```python
from build123d import *

# Parameters (mm, degrees)
F1_DEPTH = 0.5


# Not quite as in the source:
# - a pattern or mirror of a feature is missing from the dataset's text; its kind, count and spacing are read off the source's solid


with BuildPart() as f1:
    # F0 (on Top) → F1 (new body)
    with BuildSketch(Plane.XY):
        Polygon((160, 0), (0, 0), (0, -1), (0, -160), (160, -160), align=None)
        Polygon((1, -1.7071067812), (1, -1), (1.7071067812, -1), (79.5, -1), (80, -1), (80.5, -1), (158.2928932188, -1), (159, -1), (159, -1.7071067812), (159, -79.5), (159, -80.5), (159, -158.2928932188), (159, -159), (158.2928932188, -159), (80.5, -159), (80, -159), (79.5, -159), (1.7071067812, -159), (1, -159), (1, -158.2928932188), (1, -80.5), (1, -80), (1, -79.5), align=None, mode=Mode.SUBTRACT)
        Polygon((78.7928932188, -79.5), (1, -79.5), (1, -80), (1, -80.5), (78.7928932188, -80.5), (79.2928932188, -80), align=None)
        Polygon((159, -79.5), (81.2071067812, -79.5), (80.7071067812, -80), (81.2071067812, -80.5), (159, -80.5), align=None)
        Polygon((79.5, -78.7928932188), (1.7071067812, -1), (1.3535533906, -1.3535533906), (79.5, -79.5), align=None)
        Polygon((1.3535533906, -1.3535533906), (1, -1.7071067812), (78.7928932188, -79.5), (79.5, -79.5), align=None)
        Polygon((146.2407427602, -146.2407427602), (80.5, -80.5), (80.5, -81.2071067812), (145.8871893697, -146.5942961508), align=None)
        Polygon((81.2071067812, -80.5), (80.5, -80.5), (146.2407427602, -146.2407427602), (146.5942961508, -145.8871893697), align=None)
        Polygon((80, -1), (79.5, -1), (79.5, -78.7928932188), (80, -79.2928932188), align=None)
        Polygon((80.5, -1), (80, -1), (80, -79.2928932188), (80.5, -78.7928932188), align=None)
        Polygon((80, -80.7071067812), (79.5, -81.2071067812), (79.5, -159), (80, -159), align=None)
        Polygon((80.5, -81.2071067812), (80, -80.7071067812), (80, -159), (80.5, -159), align=None)
        Polygon((146.5942961508, -145.8871893697), (146.2407427602, -146.2407427602), (158.6464466094, -158.6464466094), (159, -158.2928932188), align=None)
        Polygon((158.6464466094, -158.6464466094), (146.2407427602, -146.2407427602), (145.8871893697, -146.5942961508), (158.2928932188, -159), align=None)
        Polygon((159, -1), (158.2928932188, -1), (149.7961722435, -9.4967209753), (150.1497256341, -9.8502743659), align=None)
        Polygon((159, -1.7071067812), (159, -1), (150.1497256341, -9.8502743659), (150.5032790247, -10.2038277565), align=None)
        Polygon((80, -79.2928932188), (79.5, -78.7928932188), (79.5, -79.5), (79.7928932188, -79.5), align=None)
        Polygon((79.5, -79.5), (78.7928932188, -79.5), (79.2928932188, -80), (79.5, -79.7928932188), align=None)
        Polygon((80.5, -78.7928932188), (80, -79.2928932188), (80.2071067812, -79.5), (80.5, -79.5), align=None)
        Polygon((79.5, -80.2071067812), (79.2928932188, -80), (78.7928932188, -80.5), (79.5, -80.5), align=None)
        Polygon((80, -80), (79.6464466094, -79.6464466094), (79.5, -79.7928932188), (79.5, -80.2071067812), (79.6464466094, -80.3535533906), align=None)
        Polygon((80.3535533906, -79.6464466094), (80, -80), (80.3535533906, -80.3535533906), (80.5, -80.2071067812), (80.5, -79.7928932188), align=None)
        Polygon((81.2071067812, -79.5), (80.5, -79.5), (80.5, -79.7928932188), (80.7071067812, -80), align=None)
        Polygon((79.7928932188, -80.5), (79.5, -80.5), (79.5, -81.2071067812), (80, -80.7071067812), align=None)
        Polygon((80.5, -80.5), (80.2071067812, -80.5), (80, -80.7071067812), (80.5, -81.2071067812), align=None)
        Polygon((80.7071067812, -80), (80.5, -80.2071067812), (80.5, -80.5), (81.2071067812, -80.5), align=None)
        Polygon((1.7071067812, -1), (1, -1), (1.3535533906, -1.3535533906), align=None)
        Polygon((1.3535533906, -1.3535533906), (1, -1), (1, -1.7071067812), align=None)
        Polygon((1.3535533906, -158.6464466094), (1, -158.2928932188), (1, -159), align=None)
        Polygon((1.3535533906, -158.6464466094), (1, -159), (1.7071067812, -159), align=None)
        Polygon((159, -158.2928932188), (158.6464466094, -158.6464466094), (159, -159), align=None)
        Polygon((159, -159), (158.6464466094, -158.6464466094), (158.2928932188, -159), align=None)
        Polygon((80, -79.5), (79.7928932188, -79.5), (79.6464466094, -79.6464466094), (80, -80), align=None)
        Polygon((80.2071067812, -79.5), (80, -79.5), (80, -80), (80.3535533906, -79.6464466094), align=None)
        Polygon((80.3535533906, -80.3535533906), (80, -80), (80, -80.5), (80.2071067812, -80.5), align=None)
        Polygon((80, -80.5), (80, -80), (79.6464466094, -80.3535533906), (79.7928932188, -80.5), align=None)
        Polygon((79.5, -79.7928932188), (79.2928932188, -80), (79.5, -80.2071067812), align=None)
        Polygon((80.7071067812, -80), (80.5, -79.7928932188), (80.5, -80.2071067812), align=None)
        Polygon((79.7928932188, -79.5), (79.5, -79.5), (79.6464466094, -79.6464466094), align=None)
        Polygon((79.6464466094, -79.6464466094), (79.5, -79.5), (79.5, -79.7928932188), align=None)
        Polygon((80.2071067812, -79.5), (80, -79.2928932188), (80, -79.5), align=None)
        Polygon((80, -79.5), (80, -79.2928932188), (79.7928932188, -79.5), align=None)
        Polygon((80.5, -79.5), (80.2071067812, -79.5), (80.3535533906, -79.6464466094), align=None)
        Polygon((79.6464466094, -80.3535533906), (79.5, -80.2071067812), (79.5, -80.5), align=None)
        Polygon((80.5, -79.7928932188), (80.5, -79.5), (80.3535533906, -79.6464466094), align=None)
        Polygon((79.6464466094, -80.3535533906), (79.5, -80.5), (79.7928932188, -80.5), align=None)
        Polygon((80, -80.7071067812), (80, -80.5), (79.7928932188, -80.5), align=None)
        Polygon((80.2071067812, -80.5), (80, -80.5), (80, -80.7071067812), align=None)
        Polygon((80.5, -80.5), (80.3535533906, -80.3535533906), (80.2071067812, -80.5), align=None)
        Polygon((80.5, -80.2071067812), (80.3535533906, -80.3535533906), (80.5, -80.5), align=None)
    extrude(amount=F1_DEPTH)

    # F1_copies: F1 across plane


with BuildPart() as f1_1:
    add(f1.part)
    add(f1.part.mirror(Plane(origin=(80, 0, 0), x_dir=(0, 0, 1), z_dir=(1, 0, 0))))


solid = f1_1.part
```
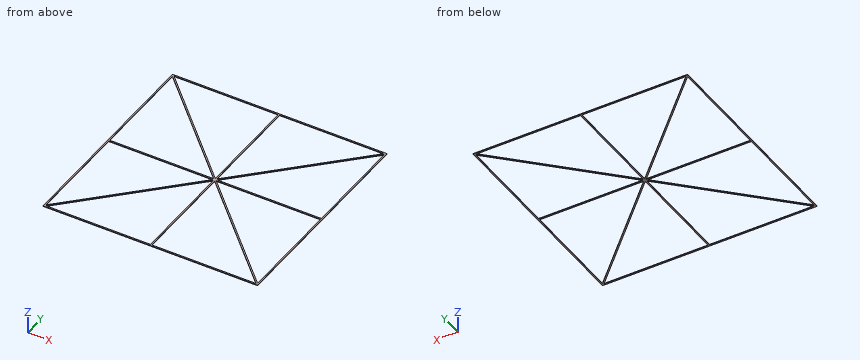
Model file for the job. Use its own axes, mm. Coordinates: 2 decimals unless noted, no trailing zeros. Loops run counter-clockwise (first coordinate to the right, second up) from the corner with the lowest first, then second, coordinate; pieces in that order, holes last. Notation, with made-up numbers: (13, 79) - (18, 79) arc R18 cw to (18, 98) - close; hole circle Ø5 at (-23.5, 61.5). An arc over 180 degrees is marked (long way). Answer as a JSON object with one key per item and string values. Group by question number.
(1) Cut at A-A (y = -87). Give the cut face in (x, z).
(2) Cut at B-B (x = 18). Give the cut face in (y, z).
(3) Cut at C-C (z = 0.4). State how many separate pieces and enclosed holes the cut face has, then the cut area to 3 significant figures.
(4) Probe line 1 along Y through (x, z) = (16.5, 0.05); line 2 along Y through (x, z) = (32, 0.45); line 3 along X through (y, z) = (-86, 0.2). List the from-to ranges inside material, lowest first.
Geometry says:
{
 "1": {"outline": "(0, 0) - (1, 0) - (1, 0.5) - (0, 0.5) - close; (72.29, 0) - (73.71, 0) - (73.71, 0.5) - (72.29, 0.5) - close; (79.5, 0) - (80.5, 0) - (80.5, 0.5) - (79.5, 0.5) - close; (86.29, 0) - (87.71, 0) - (87.71, 0.5) - (86.29, 0.5) - close; (159, 0) - (160, 0) - (160, 0.5) - (159, 0.5) - close"},
 "2": {"outline": "(-160, 0) - (-159, 0) - (-159, 0.5) - (-160, 0.5) - close; (-142.71, 0) - (-141.29, 0) - (-141.29, 0.5) - (-142.71, 0.5) - close; (-80.5, 0) - (-79.5, 0) - (-79.5, 0.5) - (-80.5, 0.5) - close; (-18.71, 0) - (-17.29, 0) - (-17.29, 0.5) - (-18.71, 0.5) - close; (-1, 0) - (0, 0) - (0, 0.5) - (-1, 0.5) - close"},
 "3": {"separate pieces": "1", "enclosed holes": "8", "area": "1,390 mm^2"},
 "4": {"line 1": "y = -160 to -159, -144.21 to -142.79, -80.5 to -79.5, -17.21 to -15.79, -1 to 0", "line 2": "y = -160 to -159, -128.71 to -127.29, -80.5 to -79.5, -32.71 to -31.29, -1 to 0", "line 3": "x = 0 to 1, 73.29 to 74.71, 79.5 to 80.5, 85.29 to 86.71, 159 to 160"}
}
